```python
from build123d import *

# Parameters (mm, degrees)
SKETCH1_W           = 1.6
SKETCH1_H           = 22
BOSS_EXTRUDE1_DEPTH = 32
SKETCH2_R           = 9.9
BOSS_EXTRUDE2_DEPTH = 6
SKETCH3_R           = 9
BOSS_EXTRUDE3_DEPTH = 10
SKETCH4_W           = 6
SKETCH4_H           = 6
BOSS_EXTRUDE4_DEPTH = 6


with BuildPart() as part:
    # Sketch1 → Boss-Extrude1 (new body)
    with BuildSketch(Plane.XY.offset(9)):
        with Locations((30, -121.5)):
            Rectangle(SKETCH1_W, SKETCH1_H)
    extrude(amount=BOSS_EXTRUDE1_DEPTH)

    # Sketch2 → Boss-Extrude2 (add)
    with BuildSketch(Plane(origin=(30.8, 0, 0), x_dir=(0, 0, -1), z_dir=(1, 0, 0))):
        with Locations((-25, -121.5)):
            Circle(SKETCH2_R)
    extrude(amount=BOSS_EXTRUDE2_DEPTH)

    # Sketch3 → Boss-Extrude3 (add)
    with BuildSketch(Plane(origin=(36.8, 0, 0), x_dir=(0, 0, -1), z_dir=(1, 0, 0))):
        with Locations((-25, -121.5)):
            Circle(SKETCH3_R)
    extrude(amount=BOSS_EXTRUDE3_DEPTH)

    # Sketch4 → Boss-Extrude4 (add)
    with BuildSketch(Plane.XY.offset(29)):
        with Locations((26.2, -116.5)):
            Rectangle(SKETCH4_W, SKETCH4_H)
    extrude(amount=BOSS_EXTRUDE4_DEPTH)


solid = part.part
```
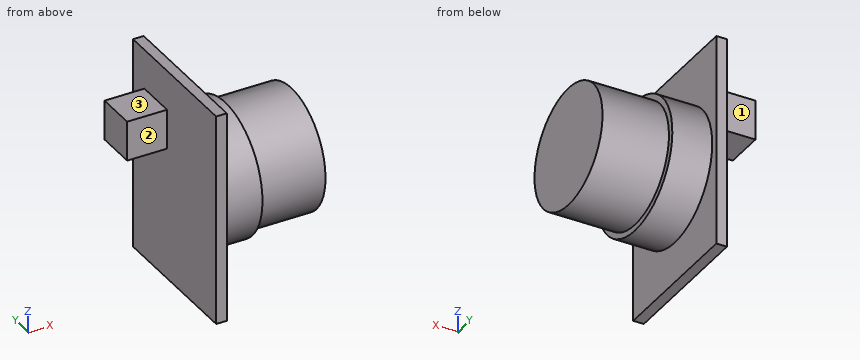
Build history of the part. All positions in model axes, mm. Face numbers are marked on the shaded views. A direction names the side the tool comes from. Round coordinates to 2 decimals unless told otherwise and drop trailing zeros. Loops run counter-clockwise (first coordinate to the right, second up) from the corner with the lowest first, then second, coordinate; pieces in that order, holes last.
Item 1: Pin check, flat tips, straight feed: P1, Ø11, axis at y = -117.5, z = 22, coming from the -X side; P2, Ø1.5, axis at y = -122, z = 15.5, coming from the +X side; P3, Ø1.8, axis at x = 24.5, y = -115.5, coming from the +Z side; P4, Ø12, axis at x = 43, y = -116.5, coming from the -Z side. Stop position of each tip, or through.
Item 2: Saw through at C-C (x = 40.5). List the corners of the cut face in (y, z), then the cut area to 3 significant figures.
Item 3: Saw through at B-B (z = 25). List the corners of the cut face in (x, y).
Item 4: Drill centre lines: line 1 along X through (y, z) = (-128, 18); line 2 along X through (y, z) = (-122.25, 36); line 3 along Z through (x, y) = (28.75, -115.25). Where is each one in solid material? Low to high.
Item 5: Saw through at A-A (y = -121.5). List the corners of the cut face in (x, z), then the cut area to 3 significant figures.
Item 6: Saw through at D-D (y = -116). List the corners of the cut face in (x, z), then the cut area to 3 significant figures.
Item 7: Which spindle directions (+Z, -Z, +X, -X, +Y, -Y) get a long thin tool onto all of the face, cutting with end or side? Do the marked faces 1, 2 and 3. Say none if no direction does.
Worked answers:
1. P1: stops at x = 29.2
1. P2: stops at x = 46.8
1. P3: stops at z = 35
1. P4: stops at z = 16
2. outline: circle Ø18 at (-121.5, 25)
2. area: 254 mm2
3. outline: (29.2, -132.5) - (30.8, -132.5) - (30.8, -131.4) - (36.8, -131.4) - (36.8, -130.5) - (46.8, -130.5) - (46.8, -112.5) - (36.8, -112.5) - (36.8, -111.6) - (30.8, -111.6) - (30.8, -110.5) - (29.2, -110.5) - close
4. line 1: x = 29.2 to 36.8
4. line 2: x = 29.2 to 30.8
4. line 3: z = 29 to 35
5. outline: (29.2, 9) - (30.8, 9) - (30.8, 15.1) - (36.8, 15.1) - (36.8, 16) - (46.8, 16) - (46.8, 34) - (36.8, 34) - (36.8, 34.9) - (30.8, 34.9) - (30.8, 41) - (29.2, 41) - close
5. area: 350 mm2
6. outline: (23.2, 29) - (29.2, 29) - (29.2, 9) - (30.8, 9) - (30.8, 16.77) - (36.8, 16.77) - (36.8, 17.88) - (46.8, 17.88) - (46.8, 32.12) - (36.8, 32.12) - (36.8, 33.23) - (30.8, 33.23) - (30.8, 41) - (29.2, 41) - (29.2, 35) - (23.2, 35) - close
6. area: 328 mm2
7. face 1: +Z, -Z, -X, +Y
7. face 2: +Z, -Z, -X, -Y
7. face 3: +Z, -X, +Y, -Y
